Model file for the job. Use its own axes, mm. A direction names the side the tool comes from. Coordinates: 2 decimals unless noted, no trailing zeros. Order: outer loops, then holes, each group sorted by start corner. A loop starts at its lowest first (then second) coordinate and runs counter-clockwise, first axis right, second up. Notation, with made-up numbers: (19, -26.5) -> (25, -26.5) arc R17 cw to (25, -2.5) -> close; hole circle Ø4 at (10, -22.5). An arc over 180 degrees is marked (long way). Write item = value, one per line. Start each with the question number.
Q1. 3-axis set-ups, long thin cutter, end or side, ignore diameter. For faces 1 (the face through (-5.75, -0.1, 1.5)), 2 (the face through (-4.75, -0.1, 1.5)), 3 (the face through (5.24, 3.24, 1.51)), 4 (the face through (-5.26, -3.24, 1.51)): which of +Z, -Z, +X, -X, +Y, -Y reach the whole face in a straight line?
Q2. Mould opens along X. For faces 5 (the face through (-1.55, 0, 1)), 6 (the face through (-2, -0.1, 1.5)), 7 (the face through (0, 6, 1.7)), 8 (the face through (-6.715, 0.084, 0.301)) say: +X half, -X half, draft (parallel to the pull), parting line (faces both ways), or undercut.
Q3. Flat gauge pin, fed straight in: pin 1 (0.8 mm diameter, centred on y = -1.5, z = 1.5, fed in from +X). Where does the tip first touch, or does it go through?
Q4. Cut at A-A, the plane z = 1.7. List the corners of the cut face in (x, y).
Q5. Cut at D-D, the plane z = 0.2. List the corners of the cut face in (x, y).
Q6. Wall check: line 1 (X direction, y = 1, z = 1.65); line 2 (X direction, y = 0.5, z = 1.35); line 3 (Z direction, x = 6, y = -4.25). Give the ranges that are in metal, low to high. Write a range as from..to.
from build123d import *

# Parameters (mm, degrees)
SKETCH1_W           = 14
SKETCH1_H           = 12
BOSS_EXTRUDE1_DEPTH = 1
SKETCH2_W           = 4
SKETCH2_H           = 12
BOSS_EXTRUDE2_DEPTH = 1
SKETCH3_W           = 3.1
SKETCH3_H           = 1.51
CUT_EXTRUDE1_DEPTH  = 15.035668848
SKETCH6_W           = 1
SKETCH6_H           = 9.5
BOSS_EXTRUDE5_DEPTH = 1
FILLET2_R           = 1
SKETCH7_W           = 1
SKETCH7_H           = 1
CUT_EXTRUDE2_DEPTH  = 1
CHAMFER1_SIZE       = 1


with BuildPart() as part:
    # Sketch1 → Boss-Extrude1 (new body)
    with BuildSketch(Plane.XY):
        Rectangle(SKETCH1_W, SKETCH1_H)
    extrude(amount=BOSS_EXTRUDE1_DEPTH)

    # Sketch2 → Boss-Extrude2 (add)
    with BuildSketch(Plane.XY.offset(1)):
        Rectangle(SKETCH2_W, SKETCH2_H)
    extrude(amount=BOSS_EXTRUDE2_DEPTH)

    # Sketch3 → Cut-Extrude1 (cut, through all)
    with BuildSketch(Plane(origin=(0, 6, 0), x_dir=(1, 0, 0), z_dir=(0, 1, 0))):
        with Locations((0, -0.755)):
            Rectangle(SKETCH3_W, SKETCH3_H)
    extrude(amount=-CUT_EXTRUDE1_DEPTH, mode=Mode.SUBTRACT)

    # Sketch6 → Boss-Extrude5 (add)
    with BuildSketch(Plane.XY.offset(1)):
        with Locations((5.25, 0)):
            Rectangle(SKETCH6_W, SKETCH6_H)
        with Locations((-5.25, 0)):
            Rectangle(SKETCH6_W, SKETCH6_H)
    extrude(amount=BOSS_EXTRUDE5_DEPTH)

    # Fillet2
    fillet2_edges = [part.edges().sort_by_distance(p)[0] for p in [
        (-4.275, 6, 0),
        (4.275, 6, 0),
        (7, 0, 0),
        (-7, 0, 0),
    ]]
    fillet(fillet2_edges, radius=FILLET2_R - 0.0001)  # a hair under: the kernel refuses the full size

    # Sketch7 → Cut-Extrude2 (cut)
    with BuildSketch(Plane.XY.offset(2)):
        with Locations((-5.25, -4.25)):
            Rectangle(SKETCH7_W, SKETCH7_H)
        with Locations((5.25, -4.25)):
            Rectangle(SKETCH7_W, SKETCH7_H)
        with Locations((-5.25, 4.25)):
            Rectangle(SKETCH7_W, SKETCH7_H)
        with Locations((5.25, 4.25)):
            Rectangle(SKETCH7_W, SKETCH7_H)
    extrude(amount=-CUT_EXTRUDE2_DEPTH, mode=Mode.SUBTRACT)

    # Chamfer1
    chamfer1_edges = [part.edges().sort_by_distance(p)[0] for p in [
        (5.25, -3.75, 2),
        (-5.25, -3.75, 2),
        (5.25, 3.75, 2),
        (-5.25, 3.75, 2),
    ]]
    chamfer(chamfer1_edges, length=CHAMFER1_SIZE - 0.0001)  # a hair under: the kernel refuses the full size


solid = part.part
Here are the results:
q1.face_1 = +Z, -X, +Y, -Y
q1.face_2 = +Z, +Y, -Y
q1.face_3 = +Z, +X, +Y
q1.face_4 = +Z, -X, -Y
q2.face_5 = undercut
q2.face_6 = undercut
q2.face_7 = draft
q2.face_8 = -X half
q3.pin_1 = 5.75
q4.outline = (-5.75, -3.05) -> (-4.75, -3.05) -> (-4.75, 3.05) -> (-5.75, 3.05) -> close; (-2, -6) -> (2, -6) -> (2, 6) -> (-2, 6) -> close; (4.75, -3.05) -> (5.75, -3.05) -> (5.75, 3.05) -> (4.75, 3.05) -> close
q5.outline = (-6.6, -6) -> (-1.55, -6) -> (-1.55, 5.6) -> (-6.6, 5.6) -> close; (1.55, -6) -> (6.6, -6) -> (6.6, 5.6) -> (1.55, 5.6) -> close
q6.line_1 = -5.75..-4.75, -2..2, 4.75..5.75
q6.line_2 = -5.75..-4.75, -2..-1.55, 1.55..2, 4.75..5.75
q6.line_3 = 0..1
